Part model, mm, in its own coordinate system. A direction names the side the tool comes from. Round coordinates to 2 decimals unless told otherwise and drop trailing zeros. Loops run counter-clockwise (first coordinate to the right, second up) from the corner with the lowest first, then second, coordinate; pieces in that order, holes last.
from build123d import *

# Parameters (mm, degrees)
F1_DEPTH = 3


# Not quite as in the source:
# - ends of sketch curves that miss each other by under 0.0002 mm in the source are joined


with BuildPart() as f1:
    # F0 (on Right) → F1 (new body)
    with BuildSketch(Plane.YZ):
        Polygon((5.5, 17.5), (-5.5, 17.5), (-16.5, 17.5), (-16.5, -17.5), (-5.5, -17.5), (5.5, -17.5), (16.5, -17.5), (16.5, 17.5), align=None)
        with BuildLine():
            Line((-16.4417464987, 2.5009048043), (-16.4935827024, 2.5))
            Line((-16.4935827024, 2.5), (-16.4660868868, 2.5078842983))
            Line((-16.4660868868, 2.5078842983), (1.1696009604, 7.5648364131))
            ThreePointArc((1.1696009604, 7.5648364131), (2.2837405131, 9.5747973722), (4.2937014722, 8.4606578195))
            ThreePointArc((4.2937014722, 8.4606578195), (4.8975775667, 5.6682772997), (5.1283712007, 2.8206836482))
            ThreePointArc((5.1283712007, 2.8206836482), (4.9431713186, -0.3431878735), (4.2978712002, -3.4460848682))
            ThreePointArc((4.2978712002, -3.4460848682), (2.2879051371, -4.5602229624), (1.1737655844, -2.5502620033))
            Line((1.1737655844, -2.5502620033), (-16.4417464987, 2.5009048043))
        make_face(mode=Mode.SUBTRACT)
        with BuildLine():
            Line((-5.5, -17.5), (-16.5, -17.5))
            Line((-16.5, -17.5), (-16.5, -21.2516473165))
            ThreePointArc((-16.5, -21.2516473165), (-16.1333008707, -22.1344656985), (-15.25, -22.5))
            Line((-15.25, -22.5), (-6.75, -22.5))
            ThreePointArc((-6.75, -22.5), (-5.8666991293, -22.1344656985), (-5.5000010855, -21.251647315))
            Line((-5.5000010855, -21.251647315), (-5.5, -17.5))
        make_face()
        with BuildLine():
            Line((16.5, -21.2516473165), (16.5, -17.5))
            Line((16.5, -17.5), (5.5, -17.5))
            Line((5.5, -17.5), (5.5, -21.251647316))
            ThreePointArc((5.5, -21.251647316), (5.8890966799, -22.1579284387), (6.8141527576, -22.5))
            Line((6.8141527576, -22.5), (15.3141527576, -22.5))
            ThreePointArc((15.3141527576, -22.5), (16.1562811226, -22.1125506362), (16.5, -21.2516473165))
        make_face()
        with BuildLine():
            Line((5.5, 18.75), (5.5, 17.5))
            Line((5.5, 17.5), (16.5, 17.5))
            Line((16.5, 17.5), (16.5, 18.75))
            ThreePointArc((16.5, 18.75), (16.1338834765, 19.6338834765), (15.25, 20))
            Line((15.25, 20), (6.75, 20))
            ThreePointArc((6.75, 20), (5.8661165235, 19.6338834765), (5.5, 18.75))
        make_face()
        with BuildLine():
            Line((-16.5, 17.5), (-5.5, 17.5))
            Line((-5.5, 17.5), (-5.5, 18.75))
            ThreePointArc((-5.5, 18.75), (-5.8661165235, 19.6338834765), (-6.75, 20))
            Line((-6.75, 20), (-15.25, 20))
            ThreePointArc((-15.25, 20), (-16.1338834765, 19.6338834765), (-16.5, 18.75))
            Line((-16.5, 18.75), (-16.5, 17.5))
        make_face()
        with BuildLine():
            Line((-16.4660868868, 2.5078842983), (-16.4417464987, 2.5009048043))
            Line((-16.4417464987, 2.5009048043), (1.8783712007, 2.8206836482))
            ThreePointArc((1.8783712007, 2.8206836482), (1.6794064974, 5.2159796384), (1.1696009604, 7.5648364131))
            Line((1.1696009604, 7.5648364131), (-16.4660868868, 2.5078842983))
        make_face()
        with BuildLine():
            Line((1.8783712007, 2.8206836482), (-16.4417464987, 2.5009048043))
            Line((-16.4417464987, 2.5009048043), (1.1737655844, -2.5502620033))
            ThreePointArc((1.1737655844, -2.5502620033), (1.7250108073, 0.1091116575), (1.8783712007, 2.8206836482))
        make_face()
    extrude(amount=F1_DEPTH)


solid = f1.part
1) Tool access for faces 5 (the face through (1, -5.5, 18)), 6 (the face through (1, 16.5, -2)), 7 (the face through (1, 0, -17.5)), 8 (the face through (1.479, 1.684, 5.183)): list every direction of +Z, -Z, +X, -X, +Y, -Y with a clear straight run to the whole face (end or side of a thin tool).
Values:
face 5: +Z, +X, -X
face 6: +Z, -Z, +X, -X, +Y
face 7: -Z, +X, -X
face 8: +X, -X
2) Slice it at C-C, the plane z = -0.5. Give the cut face in (x, y).
Values:
outline: (0, -16.5) - (3, -16.5) - (3, 1.63) - (0, 1.63) - close; (0, 4.92) - (3, 4.92) - (3, 16.5) - (0, 16.5) - close
3) Wall check: line 1 along Y through (x, z) = (1.7, -21); line 2 along Z through (x, y) = (1.65, -14); line 3 along Z through (x, y) = (2.85, -4.5). Give the ranges that are in metal, low to high.
Values:
line 1: y = -16.5 to -5.5, 5.5 to 16.5
line 2: z = -22.5 to 20
line 3: z = -17.5 to 17.5
4) Mould opens along Y. For faces 1 (the face through (1.479, -16.143, -22.125)), 2 (the face through (0, 0, -1)), 3 (the face through (1.479, 5.876, 19.644)), 4 (the face through (1.48, 16.15, -22.12)) say: released by +Y, released by -Y, zero draft, split by the parting line, or undercut.
Values:
face 1: released by -Y
face 2: zero draft
face 3: undercut
face 4: released by +Y
5) Slice it at A-A, the plane z = -18. Give the cut face in (x, y).
Values:
outline: (0, -16.5) - (3, -16.5) - (3, -5.5) - (0, -5.5) - close; (0, 5.5) - (3, 5.5) - (3, 16.5) - (0, 16.5) - close
6) Drop flat-ended pins along their axis: pin 1 Ø0.9 at (x, y) = (1, -0.5) entering from +Z; pin 2 Ø1.5 at (x, y) = (1.5, -2.5) entering from -Z. Give the stop position or say it passes through.
Values:
pin 1: stops at z = 17.5
pin 2: stops at z = -17.5
